Drawing for the job (mm, zero at the part's lowest x, y, z). A direction names the side the tool comes from. Round coordinates to 2 decimals unless told otherwise and drop trailing zeros. Order: outer loops, then holes, each group sorted by start corner. A loop starts at its lowest first (then second) coordinate and runs counter-clockwise, first axis right, second up. Notation, with made-up numbers: (16, 10.5) - (51, 10.5) arc R12 ccw to (51, 27.5) - close; hole circle Ø2 at (35, 19.25). An arc over 180 degrees is marked (long way). Answer as a JSON object with one key per item and string values.
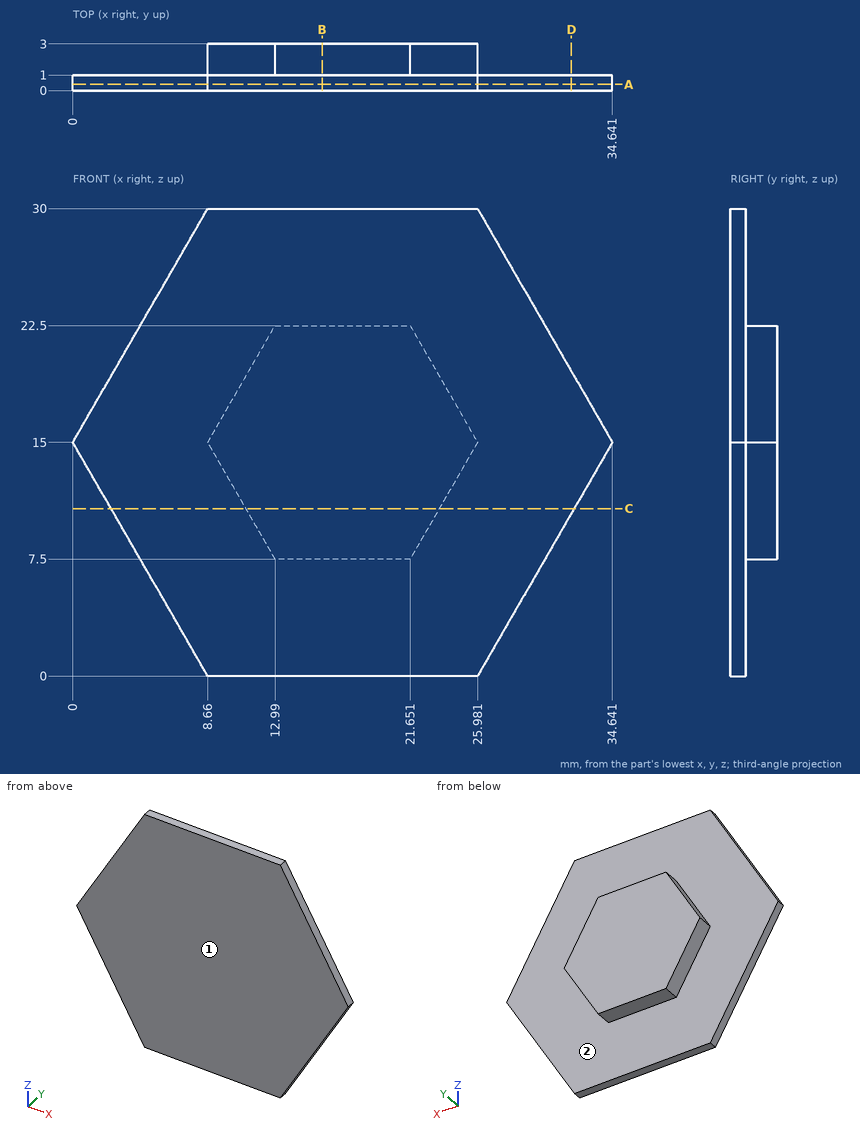
Item 1: Probe L1, parallel to Y at x = 5, z = 15.5; L2, parallel to Z at x = 18, y = 2.5; L3, parallel to X at y = 1.1, z = 18.75 (1 decimal). List the from-to ranges inside material, lowest first. Write a range as from..to.
Taken from the geometry:
{"L1": "0..1", "L2": "7.5..22.5", "L3": "10.8..23.8"}
Item 2: Drop flat-ended pins along their axis: P1, Ø1.6, axis at x = 18.5, y = 2.5, coming from the +Z side; P2, Ø0.6, axis at x = 16, y = 2, coming from the -Z side; P3, Ø1.5, axis at x = 27, z = 18.5, coming from the +Y side. Give the stop position or say it passes through.
Taken from the geometry:
{"P1": "z = 22.5", "P2": "z = 7.5", "P3": "y = 1"}
Item 3: Tool access for the marked faces 1 and 2: list every direction of +Z, -Z, +X, -X, +Y, -Y with a clear straight run to the whole face (end or side of a thin tool).
Taken from the geometry:
{"face 1": "+Z, -Z, +X, -X, -Y", "face 2": "+Y"}
Item 4: Cut at D-D (x = 32). Write the cut outline in (y, z) (1 decimal).
Taken from the geometry:
{"outline": "(0, 10.4) - (1, 10.4) - (1, 19.6) - (0, 19.6) - close"}
Item 5: Cut at C-C (z = 10.75). Write the cut outline in (x, y).
Taken from the geometry:
{"outline": "(2.45, 0) - (32.19, 0) - (32.19, 1) - (23.53, 1) - (23.53, 3) - (11.11, 3) - (11.11, 1) - (2.45, 1) - close"}
Item 6: Cut at B-B (x = 16). Write the cut outline in (y, z).
Taken from the geometry:
{"outline": "(0, 0) - (1, 0) - (1, 7.5) - (3, 7.5) - (3, 22.5) - (1, 22.5) - (1, 30) - (0, 30) - close"}
Item 7: Cut at A-A (y = 0.4). Write the cut outline in (x, z).
Taken from the geometry:
{"outline": "(0, 15) - (8.66, 0) - (25.98, 0) - (34.64, 15) - (25.98, 30) - (8.66, 30) - close"}
